from build123d import *
from OCP.BRepFilletAPI import BRepFilletAPI_MakeChamfer

# Parameters (mm, degrees)
SALIENTE_EXTRUIR2_DEPTH = 50
CHAFL_N1_SIZE           = 0.5
CHAFL_N1_SIZE2          = 0.866025404


with BuildPart() as part:
    # Croquis1 → Saliente-Extruir2 (new body)
    with BuildSketch(Plane(origin=(0, 0, 0), x_dir=(1, 0, 0), z_dir=(0, 1, 0))):
        with BuildLine():
            Line((-5.5, 4), (-7.5, 2))
            Line((-7.5, 2), (-9.5, 4))
            Line((-9.5, 4), (-9.5, 7))
            ThreePointArc((-9.5, 7), (-9.207106781, 7.707106781), (-8.5, 8))
            Line((-8.5, 8), (8.5, 8))
            ThreePointArc((8.5, 8), (9.207106781, 7.707106781), (9.5, 7))
            Line((9.5, 7), (9.5, -7))
            ThreePointArc((9.5, -7), (9.207106781, -7.707106781), (8.5, -8))
            Line((8.5, -8), (-8.5, -8))
            ThreePointArc((-8.5, -8), (-9.207106781, -7.707106781), (-9.5, -7))
            Line((-9.5, -7), (-9.5, -4))
            Line((-9.5, -4), (-7.5, -2))
            Line((-7.5, -2), (-5.5, -4))
            Line((-5.5, -4), (5.5, -4))
            Line((5.5, -4), (5.5, 4))
            Line((5.5, 4), (-5.5, 4))
        make_face()
    extrude(amount=SALIENTE_EXTRUIR2_DEPTH)

    # Chaflán1: one chamfer whose edges measure the first distance from different faces: ONE call of the kernel's chamfer builder (chamfer() names one face for all edges)
    chafl_n1_edges_1 = [part.edges().sort_by_distance(p)[0] for p in [
        (0, 50, 4),
    ]]
    chafl_n1_side_1 = [part.faces().sort_by_distance(p)[0] for p in [
        (0, 25, 4),
    ]]
    chafl_n1_edges_2 = [part.edges().sort_by_distance(p)[0] for p in [
        (-6.5, 50, 3),
    ]]
    chafl_n1_side_2 = [part.faces().sort_by_distance(p)[0] for p in [
        (-6.5, 25, 3),
    ]]
    chafl_n1_edges_3 = [part.edges().sort_by_distance(p)[0] for p in [
        (-6.5, 0, -3),
        (-8.5, 0, -3),
        (-9.5, 0, -5.5),
        (-9.207106781, 0, -7.707106781),
        (0, 0, -8),
        (9.207106781, 0, -7.707106781),
        (9.5, 0, 0),
        (9.207106781, 0, 7.707106781),
        (0, 0, 8),
        (-9.207106781, 0, 7.707106781),
        (-9.5, 0, 5.5),
        (-8.5, 0, 3),
        (-6.5, 0, 3),
        (0, 0, 4),
        (5.5, 0, 0),
        (0, 0, -4),
    ]]
    chafl_n1_side_3 = [part.faces().sort_by_distance(p)[0] for p in [
        (-9.0314651, 0, 7.5314651),
    ]]
    chafl_n1_edges_4 = [part.edges().sort_by_distance(p)[0] for p in [
        (-8.5, 50, 3),
    ]]
    chafl_n1_side_4 = [part.faces().sort_by_distance(p)[0] for p in [
        (-8.5, 25, 3),
    ]]
    chafl_n1_edges_5 = [part.edges().sort_by_distance(p)[0] for p in [
        (-9.5, 50, 5.5),
    ]]
    chafl_n1_side_5 = [part.faces().sort_by_distance(p)[0] for p in [
        (-9.5, 25, 5.5),
    ]]
    chafl_n1_edges_6 = [part.edges().sort_by_distance(p)[0] for p in [
        (-9.207106781, 50, 7.707106781),
    ]]
    chafl_n1_side_6 = [part.faces().sort_by_distance(p)[0] for p in [
        (-9.207106781, 25, 7.707106781),
    ]]
    chafl_n1_edges_7 = [part.edges().sort_by_distance(p)[0] for p in [
        (0, 50, 8),
    ]]
    chafl_n1_side_7 = [part.faces().sort_by_distance(p)[0] for p in [
        (0, 25, 8),
    ]]
    chafl_n1_edges_8 = [part.edges().sort_by_distance(p)[0] for p in [
        (9.207106781, 50, 7.707106781),
    ]]
    chafl_n1_side_8 = [part.faces().sort_by_distance(p)[0] for p in [
        (9.207106781, 25, 7.707106781),
    ]]
    chafl_n1_edges_9 = [part.edges().sort_by_distance(p)[0] for p in [
        (9.5, 50, 0),
    ]]
    chafl_n1_side_9 = [part.faces().sort_by_distance(p)[0] for p in [
        (9.5, 25, 0),
    ]]
    chafl_n1_edges_10 = [part.edges().sort_by_distance(p)[0] for p in [
        (9.207106781, 50, -7.707106781),
    ]]
    chafl_n1_side_10 = [part.faces().sort_by_distance(p)[0] for p in [
        (9.207106781, 25, -7.707106781),
    ]]
    chafl_n1_edges_11 = [part.edges().sort_by_distance(p)[0] for p in [
        (0, 50, -8),
    ]]
    chafl_n1_side_11 = [part.faces().sort_by_distance(p)[0] for p in [
        (0, 25, -8),
    ]]
    chafl_n1_edges_12 = [part.edges().sort_by_distance(p)[0] for p in [
        (0, 50, -4),
    ]]
    chafl_n1_side_12 = [part.faces().sort_by_distance(p)[0] for p in [
        (0, 25, -4),
    ]]
    chafl_n1_edges_13 = [part.edges().sort_by_distance(p)[0] for p in [
        (-9.207106781, 50, -7.707106781),
    ]]
    chafl_n1_side_13 = [part.faces().sort_by_distance(p)[0] for p in [
        (-9.207106781, 25, -7.707106781),
    ]]
    chafl_n1_edges_14 = [part.edges().sort_by_distance(p)[0] for p in [
        (-9.5, 50, -5.5),
    ]]
    chafl_n1_side_14 = [part.faces().sort_by_distance(p)[0] for p in [
        (-9.5, 25, -5.5),
    ]]
    chafl_n1_edges_15 = [part.edges().sort_by_distance(p)[0] for p in [
        (-8.5, 50, -3),
    ]]
    chafl_n1_side_15 = [part.faces().sort_by_distance(p)[0] for p in [
        (-8.5, 25, -3),
    ]]
    chafl_n1_edges_16 = [part.edges().sort_by_distance(p)[0] for p in [
        (-6.5, 50, -3),
    ]]
    chafl_n1_side_16 = [part.faces().sort_by_distance(p)[0] for p in [
        (-6.5, 25, -3),
    ]]
    chafl_n1_edges_17 = [part.edges().sort_by_distance(p)[0] for p in [
        (5.5, 50, 0),
    ]]
    chafl_n1_side_17 = [part.faces().sort_by_distance(p)[0] for p in [
        (5.5, 25, 0),
    ]]
    chafl_n1 = BRepFilletAPI_MakeChamfer(part.part.solid().wrapped)
    for e in chafl_n1_edges_1:
        chafl_n1.Add(CHAFL_N1_SIZE, CHAFL_N1_SIZE2, e.wrapped, chafl_n1_side_1[0].wrapped)  # the first distance lies on this face
    for e in chafl_n1_edges_2:
        chafl_n1.Add(CHAFL_N1_SIZE, CHAFL_N1_SIZE2, e.wrapped, chafl_n1_side_2[0].wrapped)  # the first distance lies on this face
    for e in chafl_n1_edges_3:
        chafl_n1.Add(CHAFL_N1_SIZE, CHAFL_N1_SIZE2, e.wrapped, chafl_n1_side_3[0].wrapped)  # the first distance lies on this face
    for e in chafl_n1_edges_4:
        chafl_n1.Add(CHAFL_N1_SIZE, CHAFL_N1_SIZE2, e.wrapped, chafl_n1_side_4[0].wrapped)  # the first distance lies on this face
    for e in chafl_n1_edges_5:
        chafl_n1.Add(CHAFL_N1_SIZE, CHAFL_N1_SIZE2, e.wrapped, chafl_n1_side_5[0].wrapped)  # the first distance lies on this face
    for e in chafl_n1_edges_6:
        chafl_n1.Add(CHAFL_N1_SIZE, CHAFL_N1_SIZE2, e.wrapped, chafl_n1_side_6[0].wrapped)  # the first distance lies on this face
    for e in chafl_n1_edges_7:
        chafl_n1.Add(CHAFL_N1_SIZE, CHAFL_N1_SIZE2, e.wrapped, chafl_n1_side_7[0].wrapped)  # the first distance lies on this face
    for e in chafl_n1_edges_8:
        chafl_n1.Add(CHAFL_N1_SIZE, CHAFL_N1_SIZE2, e.wrapped, chafl_n1_side_8[0].wrapped)  # the first distance lies on this face
    for e in chafl_n1_edges_9:
        chafl_n1.Add(CHAFL_N1_SIZE, CHAFL_N1_SIZE2, e.wrapped, chafl_n1_side_9[0].wrapped)  # the first distance lies on this face
    for e in chafl_n1_edges_10:
        chafl_n1.Add(CHAFL_N1_SIZE, CHAFL_N1_SIZE2, e.wrapped, chafl_n1_side_10[0].wrapped)  # the first distance lies on this face
    for e in chafl_n1_edges_11:
        chafl_n1.Add(CHAFL_N1_SIZE, CHAFL_N1_SIZE2, e.wrapped, chafl_n1_side_11[0].wrapped)  # the first distance lies on this face
    for e in chafl_n1_edges_12:
        chafl_n1.Add(CHAFL_N1_SIZE, CHAFL_N1_SIZE2, e.wrapped, chafl_n1_side_12[0].wrapped)  # the first distance lies on this face
    for e in chafl_n1_edges_13:
        chafl_n1.Add(CHAFL_N1_SIZE, CHAFL_N1_SIZE2, e.wrapped, chafl_n1_side_13[0].wrapped)  # the first distance lies on this face
    for e in chafl_n1_edges_14:
        chafl_n1.Add(CHAFL_N1_SIZE, CHAFL_N1_SIZE2, e.wrapped, chafl_n1_side_14[0].wrapped)  # the first distance lies on this face
    for e in chafl_n1_edges_15:
        chafl_n1.Add(CHAFL_N1_SIZE, CHAFL_N1_SIZE2, e.wrapped, chafl_n1_side_15[0].wrapped)  # the first distance lies on this face
    for e in chafl_n1_edges_16:
        chafl_n1.Add(CHAFL_N1_SIZE, CHAFL_N1_SIZE2, e.wrapped, chafl_n1_side_16[0].wrapped)  # the first distance lies on this face
    for e in chafl_n1_edges_17:
        chafl_n1.Add(CHAFL_N1_SIZE, CHAFL_N1_SIZE2, e.wrapped, chafl_n1_side_17[0].wrapped)  # the first distance lies on this face
    add(Compound.cast(chafl_n1.Shape()), mode=Mode.REPLACE)


solid = part.part
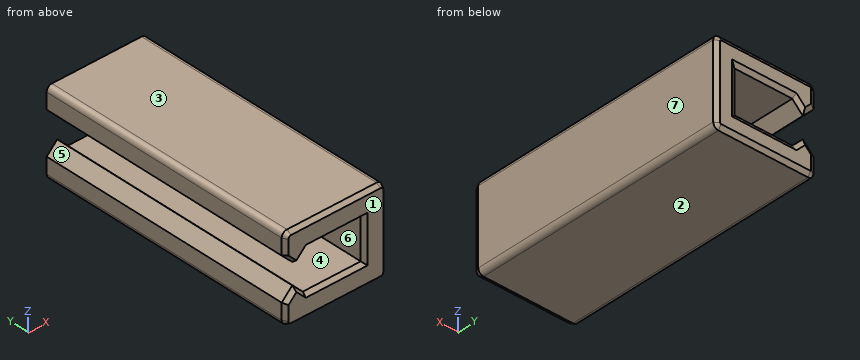
Geometry check sheet. Reference: the model listing, model coordinates, mm. Face numbers are marked on the shaded views. A direction names the side the tool comes from. Give positions to 0.01 mm unless a question says otherwise; leave off trailing zeros. Order: outer loops, then holes, each group sorted by start corner. A loop starts at its lowest first (then second) coordinate and runs counter-clockwise, first axis right, second up. Notation, with made-up numbers: (26, -10.5) - (53, -10.5) arc R22 cw to (53, 2.5) - close; hole circle Ø3 at (88.25, 22). An arc over 180 degrees is marked (long way). Use one line per item in the form item = value.
1) Depth check by flat-ended pin: pin 1 Ø4 at (x, z) = (-4, -2.5) entering from +Y; pin 2 Ø2.5 at (y, z) = (16, -1.5) entering from -X. Enter the tip coordinate at first touch or a pass-through.
Working result:
pin_1 = 49.79
pin_2 = -8.25
2) Sectioned sample at C-C (y = 45). Record the boundary of the cut face in (x, z), and give its area (3 significant figures).
Working result:
outline = (-9.5, -7) arc R1 ccw to (-8.5, -8) - (8.5, -8) arc R1 ccw to (9.5, -7) - (9.5, 7) arc R1 ccw to (8.5, 8) - (-8.5, 8) arc R1 ccw to (-9.5, 7) - (-9.5, 4) - (-7.5, 2) - (-5.5, 4) - (5.5, 4) - (5.5, -4) - (-5.5, -4) - (-7.5, -2) - (-9.5, -4) - close
area = 191 mm^2
3) Sectioned sample at B-B (z = -0.75). Record the boundary of the cut face in (x, y).
Working result:
outline = (5.5, 0.87) - (6, 0) - (9, 0) - (9.5, 0.87) - (9.5, 49.5) - (8.63, 50) - (6.37, 50) - (5.5, 49.5) - close
4) Access from +Z, -Z, +X, -X, +Y, -Y to the whole of each face (thin tool, end or side, straight path). Record for the marked faces 5, 6 and 7.
Working result:
face_5 = -X, +Y, -Y
face_6 = +Y, -Y
face_7 = +Z, -Z, +X, +Y, -Y
5) Sectioned sample at A-A (x = 3.5). Record the boundary of the cut face in (y, z).
Working result:
outline = (0, -7.5) - (0.87, -8) - (49.5, -8) - (50, -7.13) - (50, -4.87) - (49.5, -4) - (0.87, -4) - (0, -4.5) - close; (0, 4.5) - (0.87, 4) - (49.5, 4) - (50, 4.87) - (50, 7.13) - (49.5, 8) - (0.87, 8) - (0, 7.5) - close
6) Draft check along Z on the marked faces 1, 2, 3 and 4. Enter one of: released by +Z, released by -Z, zero draft, split by the parting line, or undercut.
Working result:
face_1 = zero draft
face_2 = released by -Z
face_3 = released by +Z
face_4 = undercut
7) Material ranges on probe 1 along Z at (x, y) = (4, 16); probe 2 along X at (y, z) = (16, 0.5); probe 3 along X at (y, z) = (25, -3.5), recorded low to high. Write a range as from..to.
Working result:
probe_1 = -8..-4, 4..8
probe_2 = 5.5..9.5
probe_3 = -9..-6, 5.5..9.5
